Source: CAD feature listing. Evaluate the final solid. Frame: model axes, mm. A direction names the side the tool comes from. Give positions to 0.01 mm unless a question says otherwise; leave off trailing zeros. Order: outer loops, then holes, each group sorted by start corner. A loop starts at its lowest first (then second) coordinate and runs counter-clockwise, first axis right, second up.
from build123d import *

# Parameters (mm, degrees)
F0_W     = 58
F0_H     = 10
F0_R     = 2.4
F1_DEPTH = 1.6
F2_R     = 3.255
F2_R_2   = 2.4
F3_DEPTH = 3.2
F4_R     = 4.99999


# Not quite as in the source:
# - a fillet or chamfer is up to 0.001 mm smaller than in the source, because OpenCascade refuses the exact size


with BuildPart() as f1:
    # F0 (on Top) → F1 (new body)
    with BuildSketch(Plane.XY):
        Rectangle(F0_W, F0_H)
        Circle(F0_R, mode=Mode.SUBTRACT)
    extrude(amount=-F1_DEPTH)

    # F2 (on face) → F3 (join)
    with BuildSketch(Plane.XY):
        Circle(F2_R)
        Circle(F2_R_2, mode=Mode.SUBTRACT)
    extrude(amount=F3_DEPTH)

    # F4 (radius 5 in the source; OpenCascade refuses exactly that, so slightly less here)
    f4_edges = [f1.edges().sort_by_distance(p)[0] for p in [
        (29, 5, -0.8),
        (29, -5, -0.8),
        (-29, 5, -0.8),
        (-29, -5, -0.8),
    ]]
    fillet(f4_edges, radius=F4_R)


solid = f1.part
1) Ray query, L1, parallel to Y at x = 0, z = 1.7 (3 decimals); L2, parallel to Y at x = 0, z = -0.1; L3, parallel to Z at x = -6, y = 0.5. Return the intervals inside material, ascending.
Checks:
L1: y = -3.255 to -2.4, 2.4 to 3.255
L2: y = -5 to -2.4, 2.4 to 5
L3: z = -1.6 to 0
2) Section query D-D on y = 4. Output: boundary loops of the cut face in (x, z), and give its area (3 significant figures).
Checks:
outline: (-27, -1.6) - (27, -1.6) - (27, 0) - (-27, 0) - close
area: 86.4 mm2
3) Section query B-B on y = -1. Output: boundary loops of the cut face in (x, z).
Checks:
outline: (-28.9, -1.6) - (-2.18, -1.6) - (-2.18, 3.2) - (-3.1, 3.2) - (-3.1, 0) - (-28.9, 0) - close; (2.18, -1.6) - (28.9, -1.6) - (28.9, 0) - (3.1, 0) - (3.1, 3.2) - (2.18, 3.2) - close
4) Section query A-A on x = 0. Output: boundary loops of the cut face in (y, z) (3 decimals), and give its area (3 significant figures).
Checks:
outline: (-5, -1.6) - (-2.4, -1.6) - (-2.4, 3.2) - (-3.255, 3.2) - (-3.255, 0) - (-5, 0) - close; (2.4, -1.6) - (5, -1.6) - (5, 0) - (3.255, 0) - (3.255, 3.2) - (2.4, 3.2) - close
area: 13.8 mm2
5) First-contact query: pin 1 Ø1.5 at (x, z) = (16.5, 2.5) entering from +Y; pin 2 Ø1 at (y, z) = (2.5, 1.5) entering from -X. Flat tips, straight axial feed; report the tip coordinate or a pass-through.
Checks:
pin 1: passes through
pin 2: stops at x = -2.57
6) Reachability of faces 1 (the face through (3.007, -1.247, 1.578)), 2 (the face through (-27, -4, -1)) from +Z, -Z, +X, -X, +Y, -Y: full face, straight path, thin tool, end or side. Return the list, or none.
Checks:
face 1: +Z
face 2: +Z, -Z, -X, -Y
7) Pull-direction query (X, two-part tool) for faces 3 (the face through (28, 3, -1)), 4 (the face through (1.29, 2.024, 0.766)), 5 (the face through (-0.4, 3.4, 0)); classes: +X half, -X half, draft (parallel to the pull), parting line (faces both ways), or undercut.
Checks:
face 3: +X half
face 4: undercut
face 5: draft
8) Section query C-C on z = 0.55. Output: boundary loops of the cut face in (x, y) (3 decimals).
Checks:
outline: circle Ø6.51 at (0, 0); hole circle Ø4.8 at (0, 0)
